```python
from build123d import *

# Parameters (mm, degrees)
F0_W     = 35.2
F0_H     = 35.2
F1_DEPTH = 42
F2_R     = 11
F3_DEPTH = 2
F5_DEPTH = 22
F7_D     = 2.4
F7_DEPTH = 4.5
F7_TIP   = 0.7210327428
F8_SIZE  = 4


with BuildPart() as f1:
    # F0 (on Front) → F1 (new body)
    with BuildSketch(Plane.XZ):
        Rectangle(F0_W, F0_H)
    extrude(amount=-F1_DEPTH)

    # F2 (on Front) → F3 (join)
    with BuildSketch(Plane.XZ):
        Circle(F2_R)
    extrude(amount=F3_DEPTH)

    # F4 (on face) → F5 (join)
    with BuildSketch(Plane.XZ.offset(2)):
        with BuildLine():
            Line((1.5, 2), (-1.5, 2))
            ThreePointArc((-1.5, 2), (0, -2.5), (1.5, 2))
        make_face()
    extrude(amount=F5_DEPTH)

    # F7
    with Locations(Plane.XZ):
        with Locations((-13, 13), (13, 13), (13, -13), (-13, -13)):
            Hole(F7_D / 2, depth=F7_DEPTH)
            with Locations((0, 0, -(F7_DEPTH + F7_TIP / 2))):  # 118° drill point
                Cone(0, F7_D / 2, F7_TIP, mode=Mode.SUBTRACT)

    # F8
    f8_edges = [f1.edges().sort_by_distance(p)[0] for p in [
        (-17.6, 21, 17.6),
        (-17.6, 21, -17.6),
        (17.6, 21, -17.6),
        (17.6, 21, 17.6),
    ]]
    chamfer(f8_edges, length=F8_SIZE)


solid = f1.part
```
Design review of the part built by this model. Coordinates are the model's own, in mm. A direction names the side the tool comes from. Give positions to 0.01 mm unless a question says otherwise; leave off trailing zeros. Loops run counter-clockwise (first coordinate to the right, second up) from the corner with the lowest first, then second, coordinate; pieces in that order, holes last. Notation, with made-up numbers: M 59,-26 L 86,-26 A24 ccw 86,9 Z; hole C 85.25,-12 d7. An arc over 180 degrees is marked long. Return JSON: item names as keys, results as strings. Group by question number.
Item 1: For probe 1 along Z at (x, y) = (-13, 3.3); probe 2 along Y at (x, z) = (-2, 13.5), list the stretches that pass through material, from the lowest coordinate up.
Item 2: We need section C-C (z = 0). Give the boundary of the cut face in (x, y), and give its area (3 significant figures).
Item 3: We need section B-B (x = 0). Give the boundary of the cut face in (y, z).
Item 4: Insertion check: pin 1 Ø2.5 at (x, y) = (-0.5, -10) entering from +Z; pin 2 Ø2 at (x, z) = (10.5, 13.5) entering from -Y. Each pin has a flat end and moves straight along its axis. Give the tip position at first contact, or say it passes through.
Item 5: We need section D-D (y = 28.5). Give the boundary of the cut face in (x, z).
Item 6: Mouldability with a two-part tool opening along X and no side actions: class faces 1 (the flat face through (15.6, 20.7, -15.6)), 2 (the flat face through (-17.6, 21, 0)), 3 (the conical face through (-13.15, 5.1, 13.14)) as released by +X, released by -X, zero draft, split by the parting line, or undercut.
Item 7: We need section A-A (y = 2). Give the boundary of the cut face in (x, z), and give its area (3 significant figures).
Item 8: Tool access review of faces 4 (the flat face through (0, -13, 2)), 5 (the flat face through (-15.6, 20.7, -15.6)), 6 (the cylindrical face through (-12.74, 2.28, 11.83)): name each direction out of +Z, -Z, +X, -X, +Y, -Y from which nothing blocks a thin tool from reaching the whole face with its end or side.
Output:
{
 "1": {"probe 1": "z = -17.6 to -14.2, -11.8 to 11.8, 14.2 to 17.6", "probe 2": "y = 0 to 42"},
 "2": {"outline": "M -17.6,0 L -11,0 L -11,-2 L -2.5,-2 L -2.5,-24 L 2.5,-24 L 2.5,-2 L 11,-2 L 11,0 L 17.6,0 L 17.6,42 L -17.6,42 Z", "area": "1,630 mm^2"},
 "3": {"outline": "M -24,-2.5 L -2,-2.5 L -2,-11 L 0,-11 L 0,-17.6 L 42,-17.6 L 42,17.6 L 0,17.6 L 0,11 L -2,11 L -2,2 L -24,2 Z"},
 "4": {"pin 1": "stops at z = 2", "pin 2": "stops at y = 0"},
 "5": {"outline": "M -17.6,-13.6 L -13.6,-17.6 L 13.6,-17.6 L 17.6,-13.6 L 17.6,13.6 L 13.6,17.6 L -13.6,17.6 L -17.6,13.6 Z"},
 "6": {"face 1": "released by +X", "face 2": "released by -X", "face 3": "undercut"},
 "7": {"outline": "M -17.6,-13.6 L -13.6,-17.6 L 13.6,-17.6 L 17.6,-13.6 L 17.6,13.6 L 13.6,17.6 L -13.6,17.6 L -17.6,13.6 Z; hole C -13,-13 d2.4; hole C -13,13 d2.4; hole C 13,-13 d2.4; hole C 13,13 d2.4", "area": "1,190 mm^2"},
 "8": {"face 4": "+Z, +X, -X, -Y", "face 5": "-Z, -X, +Y, -Y", "face 6": "-Y"}
}
